Work out the finished part from the listing and answer in its coordinate system (mm). Face numbers are marked on the shaded views. A direction names the side the tool comes from. Coordinates: 2 decimals unless noted, no trailing zeros. Order: outer loops, then holes, each group sorted by start corner. A loop starts at its lowest first (then second) coordinate and runs counter-clockwise, first axis right, second up. Notation, with made-up numbers: (26.25, 64.25) - (30.25, 64.25) arc R16 ccw to (30.25, 94.25) - close; hole circle Ø5 at (6.25, -13.5). An arc over 180 degrees is marked (long way). Answer as a JSON object with one key per item and string values. Group by question number.
1) Section C-C (x = 0.3) is taken. Give the vertices of the cut face in (y, z).
2) The mould has two halves that part along Z. Classify the marked faces 4, 5 and 6: released by +Z, released by -Z, zero draft, split by the parting line, or undercut.
3) Each of these flat-tipped pins is pushed along its axis until it touches: P1, Ø1.9, axis at x = -2, y = -2, coming from the -Z side; P2, Ø1.1, axis at x = -2, y = -4.5, coming from the +Z side; P3, Ø0.9, axis at x = -2, z = -1, coming from the +Y side; P4, Ø2.5, axis at y = -4.2, z = -5.2, coming from the +X side. Where does it stop, or does it pass through?
4) A tool of negligible diameter and unlimited length cuts with its end or side. For the marked faces 1, 2 and 3, from which of +Z, -Z, +X, -X, +Y, -Y can it reach the whole face along a straight path? Write none if from no direction.
5) Section B-B (z = -8) is taken. Give the vertices of the cut face in (x, y).
6) Section A-A (x = -2.7) is taken. Give the vertices of the cut face in (y, z) (1 decimal).
7) Find the intervals of material crossed by line 1 along Y through (x, z) = (-0.8, 0); line 2 along Y through (x, z) = (-2.6, -1.25); line 3 along Y through (x, z) = (0.75, -5.2), in increasing order.
Autodesk Inventor part; units mm, degrees
ref_plane "YZ Plane" through (0, 0, 0) normal (1, 0, 0) x (0, 1, 0)
ref_plane "XZ Plane" through (0, 0, 0) normal (0, 1, 0) x (-1, 0, 0)
ref_plane "XY Plane" through (0, 0, 0) normal (0, 0, 1) x (1, 0, 0)
sketch "Sketch1" plane through (0, 0, 0) normal (1, 0, 0) x (0, 1, 0)
  circle A0 centre (0, 0) radius 10
  line L0 (10, 0) -> (8.1, 0)
  circle A1 centre (8.1, 0) radius 1.5
  circle A2 centre (0, 0) radius 3
  circle A3 centre (-8.1, 0) radius 1.5
  dimension "d0" = 20
  dimension "d1" = 1.9
  dimension "d2" = 3
  dimension "d3" = 6
  dimension "d29" = 360
extrude "Extrusion1" add sketch "Sketch1" along normal blind 1
sketch "Sketch2" plane through (0, 0, 0) normal (-1, 0, 0) x (0, 0, 1)
  line L0 (0, 5.5) -> (-6.5, 5.5)
  line L1 (0, 5.5) -> (2.5, 5.5)
  line L2 (6.0478, 3.0122) -> (6.0478, -2.8019)
  line L3 (-6.5, -5.5) -> (-6.5, 5.5)
  line L4 (5.5, 5.498) -> (2.5, 5.5)
  line L5 (2.5, 5.5) -> (6.0478, 3.0122)
  line L6 (5.2, -5.498) -> (2.2, -5.5)
  line L7 (2.2, -5.5) -> (6.0478, -2.8019)
  line L8 (2.2, -5.5) -> (-6.5, -5.5)
  line L9 (2.5631, 5.7) -> (6.585, 2.8798)
  line L10 (6.585, 2.8798) -> (6.585, -2.7667)
  line L11 (6.585, -2.7667) -> (2.4018, -5.7)
  line L12 (2.5631, 5.7) -> (0, 5.7)
  line L13 (0, 5.7) -> (-6.7, 5.7)
  line L14 (-6.7, 5.7) -> (-6.7, -5.7)
  line L15 (-6.7, -5.7) -> (2.4018, -5.7)
  circle A0 centre (0, 0) radius 10
  circle A1 centre (0, 0) radius 10
  line L16 (10, 0) -> (10, 1)
  line L17 (10, 1) -> (6.585, 1)
  line L18 (10, 0) -> (10, -1)
  line L19 (10, 0) -> (11, 0) construction
  line L20 (10, -1) -> (6.585, -1)
  line L21 (-10, 0) -> (-10, 3.5)
  line L22 (-10, 3.5) -> (-6.7, 3.5)
  line L23 (-10, 0) -> (-10, -3.5)
  line L24 (-10, -3.5) -> (-6.7, -3.5)
  circle A2 centre (0, 8.1) radius 1.5
  circle A3 centre (0, 8.1) radius 1.5
  circle A4 centre (0, -8.1) radius 1.5
  point P0 (-9.3675, -3.5)
  point P1 (9.9499, -1)
  point P2 (9.9499, 1)
  point P3 (-9.3675, 3.5)
  dimension "d6" = 5.5
  dimension "d7" = 6.5
  dimension "d8" = 5.5
  dimension "d9" = 11
  dimension "d10" = 3
  dimension "d11" = 35
  dimension "d12" = 3
  dimension "d13" = 35
  dimension "d14" = 0.2
  dimension "d15" = 0.2
  dimension "d18" = 1
  dimension "d19" = 1
  dimension "d20" = 270
  dimension "d21" = 3.5
  dimension "d22" = 3.5
  dimension "d33" = 360
extrude "Extrusion2" add sketch "Sketch2" along normal blind 3 contours L9 L12 L13 L14 L22 A0 L17 L10 | L11 L10 L20 A0 L24 L14 L15
sketch "Sketch3" plane through (0, 0, 0) normal (-1, 0, 0) x (0, 0, 1)
  circle A0 centre (-5.2, 4.2) radius 1.5
  circle A1 centre (-5.2, -4.2) radius 1.5
  line L0 (-6.7, 5.7) -> (2.5631, 5.7)
  line L1 (-6.7, 3.5) -> (-6.7, 5.7)
  line L2 (-6.7, -5.7) -> (-6.7, -3.5)
  line L3 (2.4018, -5.7) -> (-6.7, -5.7)
  point P0 (0, 0)
  dimension "d23" = 3
  dimension "d24" = 3
extrude "Extrusion3" cut sketch "Sketch3" against normal blind 10 contours A0 | A1
properties part number "potentiometer_holder"
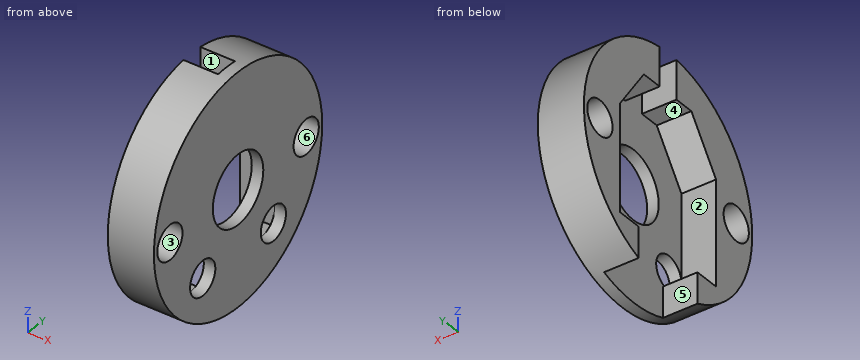
Report:
{
 "1": {"outline": "circle Ø20 at (0, 0); hole circle Ø3 at (-8.1, 0); hole circle Ø3 at (-4.2, -5.2); hole circle Ø6 at (0, 0); hole circle Ø3 at (4.2, -5.2); hole circle Ø3 at (8.1, 0)"},
 "2": {"face 4": "released by -Z", "face 5": "zero draft", "face 6": "undercut"},
 "3": {"P1": "stops at z = 6.32", "P2": "stops at z = 9.19", "P3": "stops at y = 9.98", "P4": "passes through"},
 "4": {"face 1": "+Z, -Z, -X", "face 2": "-X", "face 3": "+X, -X"},
 "5": {"outline": "(-3, -6) - (1, -6) - (1, 6) - (-3, 6) - (-3, 3.5) - (0, 3.5) - (0, -3.5) - (-3, -3.5) - close"},
 "6": {"outline": "(-5.7, -6.7) - (-5.7, 2.4) - (-2.8, 6.6) - (-1, 6.6) - (-1, 9.9) arc R10 ccw to (-3.5, -9.4) - (-3.5, -6.7) - close; (1, 6.6) - (2.9, 6.6) - (5.7, 2.6) - (5.7, -6.7) - (3.5, -6.7) - (3.5, -9.4) arc R10 ccw to (1, 9.9) - close; hole circle Ø3 at (-8.1, 0); hole circle Ø3 at (8.1, 0)"},
 "7": {"line 1": "y = -10 to -9.6, -6.6 to -5.7, 5.7 to 6.6, 9.6 to 10", "line 2": "y = -9.92 to -8.93, -7.27 to -5.7, 5.7 to 7.27, 8.93 to 9.92", "line 3": "y = -8.54 to -5.7, -2.7 to 2.7, 5.7 to 8.54"}
}
